from build123d import *

# Parameters (mm, degrees)
CUT_EXTRUDE1_DEPTH      = 34.608034754
CUT_EXTRUDE1_DEPTH_BACK = 34.608034754
SKETCH2_R               = 1.5


with BuildPart() as part:
    # Sketch1 → Revolve1 (revolve)
    with BuildSketch(Plane.XY, mode=Mode.PRIVATE) as revolve1_sk:
        Polygon((0, 15), (0, 23.5), (5, 23.5), (5, 17.5), (3, 17.5), (3, 15), align=None)
    revolve(revolve1_sk.sketch.rotate(Axis((0, 0, 0), (1, 0, 0)), 90), axis=Axis((0, 0, 0), (1, 0, 0)))

    # Sketch2 → Cut-Extrude1 (cut, two sides: drawn at the far end of the back side and taken through both)
    with BuildSketch(Plane.ZY.offset(-CUT_EXTRUDE1_DEPTH_BACK)):
        with Locations((0, 20.5)):
            Circle(SKETCH2_R)
        with Locations((17.753520778, -10.25)):
            Circle(SKETCH2_R)
        with Locations((-17.753520778, -10.25)):
            Circle(SKETCH2_R)
    extrude(amount=CUT_EXTRUDE1_DEPTH + CUT_EXTRUDE1_DEPTH_BACK, mode=Mode.SUBTRACT)


solid = part.part
Part model, mm, in its own coordinate system. A direction names the side the tool comes from. Coordinates: 2 decimals unless noted, no trailing zeros. Order: outer loops, then holes, each group sorted by start corner. A loop starts at its lowest first (then second) coordinate and runs counter-clockwise, first axis right, second up. Notation, with made-up numbers: (-12, 38.5) - (12, 38.5) arc R20 cw to (12, 66.5) - close; hole circle Ø10 at (-19, 41). An arc over 180 degrees is marked (long way). Use CSV: the item, a comma, the result in double quotes.
Item 1: Probe probe 1 along Y at (x, z) = (1.65, 0); probe 2 along Y at (x, z) = (4.25, 0); probe 3 along Z at (x, y) = (2.9, -10.25). List the from-to ranges inside material, lowest first.
Solved:
probe 1,"y = -23.5 to -15, 15 to 19, 22 to 23.5"
probe 2,"y = -23.5 to -17.5, 17.5 to 19, 22 to 23.5"
probe 3,"z = -21.15 to -19.25, -16.25 to -10.95, 10.95 to 16.25, 19.25 to 21.15"
Item 2: Saw through at C-C on x = 1.3. Give the cut face in (y, z).
Solved:
outline,"circle Ø47 at (0, 0); hole circle Ø30 at (0, 0); hole circle Ø3 at (-10.25, -17.75); hole circle Ø3 at (-10.25, 17.75); hole circle Ø3 at (20.5, 0)"
Item 3: 3-axis set-ups, long thin cutter, end or side, ignore diameter. For faces 1 (the face through (1.48, -12.65, 8.06)), 2 (the face through (3, -8, 13)): which of +Z, -Z, +X, -X, +Y, -Y reach the whole face in a straight line?
Solved:
face 1,"+X, -X"
face 2,"+X"
Item 4: Saw through at D-D on z = 9.5. Give the cut face in (x, y).
Solved:
outline,"(0, -21.49) - (5, -21.49) - (5, -14.7) - (3, -14.7) - (3, -11.61) - (0, -11.61) - close; (0, 11.61) - (3, 11.61) - (3, 14.7) - (5, 14.7) - (5, 21.49) - (0, 21.49) - close"
Item 5: Mould opens along Z. For faces 3 (the face through (0, -0.3, -15.3)), 4 (the face through (2.54, -23.3, -3.06)), 5 (the face through (2.535, -11.714, 17.428)) say: +Z half, -Z half, draft (parallel to the pull), parting line (faces both ways), or undercut.
Solved:
face 3,"draft"
face 4,"parting line"
face 5,"undercut"
Item 6: Saw through at B-B on z = 0. Give the cut face in (x, y), and give its area (3 significant figures).
Solved:
outline,"(0, -23.5) - (5, -23.5) - (5, -17.5) - (3, -17.5) - (3, -15) - (0, -15) - close; (0, 15) - (3, 15) - (3, 17.5) - (5, 17.5) - (5, 19) - (0, 19) - close; (0, 22) - (5, 22) - (5, 23.5) - (0, 23.5) - close"
area,"60.0 mm²"
Item 7: Drop flat-ended pins along their axis: P1, Ø1, axis at x = 3.5, z = -5.5, coming from the -Y side; P2, Ø1, axis at x = 1, y = 2.5, coming from the -Z side; P3, Ø2, axis at x = 2.5, y = 13.5, coming from the +Z side. Give the stop position or say it passes through.
Solved:
P1,"stops at y = -22.96"
P2,"stops at z = -23.41"
P3,"stops at z = 19.9"
Item 8: Saw through at A-A on y = 0. Give the cut face in (x, z), and give its area (3 significant figures).
Solved:
outline,"(0, -23.5) - (5, -23.5) - (5, -17.5) - (3, -17.5) - (3, -15) - (0, -15) - close; (0, 15) - (3, 15) - (3, 17.5) - (5, 17.5) - (5, 23.5) - (0, 23.5) - close"
area,"75.0 mm²"
